```python
from build123d import *

# Parameters (mm, degrees)
F0_R     = 50.8
F1_DEPTH = 6.35
F2_DEPTH = 38.1
F3_DEPTH = 63.5


with BuildPart() as f1:
    # F0 (on Front) → F1 (new body, symmetric)
    with BuildSketch(Plane.XZ):
        Circle(F0_R)
        Polygon((0, -47.0656435661), (-38.1, 18.9254922023), (38.1, 18.9254922023), align=None, mode=Mode.SUBTRACT)
    extrude(amount=F1_DEPTH, both=True)

    # F0 (on Front) → F2 (join, symmetric)
    with BuildSketch(Plane.XZ):
        with BuildLine():
            add(Edge.make_bspline(
                [(75.8723819512, 94.9205090511), (75.9331390119, 77.3418365937), (1.5317360093, 89.0560595825), (22.3357510028, 101.1633279928)],
                knots=[0, 0, 0, 0, 53.8993844273, 53.8993844273, 53.8993844273, 53.8993844273], degree=3))
            Line((22.3357510028, 101.1633279928), (-119.3492407465, 18.707214336))
            Line((-119.3492407465, 18.707214336), (-152.3990897254, -0.5267360641))
            Line((-152.3990897254, -0.5267360641), (-119.5423719358, -19.3454558368))
            Line((-119.5423719358, -19.3454558368), (76.6557116753, -131.7181151837))
            Line((76.6557116753, -131.7181151837), (76.5361384347, -97.1223199462))
            Line((76.5361384347, -97.1223199462), (25.7361384347, -97.1223199462))
            Line((25.7361384347, -97.1223199462), (25.7361384347, -71.7223199462))
            Line((25.7361384347, -71.7223199462), (76.4483485663, -71.7223199462))
            Line((76.4483485663, -71.7223199462), (75.8723819512, 94.9205090511))
        make_face()
        Circle(F0_R, mode=Mode.SUBTRACT)
        with BuildLine():
            Line((75.7433780501, 132.2448512478), (22.3357510028, 101.1633279928))
            add(Edge.make_bspline(
                [(75.8723819512, 94.9205090511), (75.9331390119, 77.3418365937), (1.5317360093, 89.0560595825), (22.3357510028, 101.1633279928)],
                knots=[0, 0, 0, 0, 53.8993844273, 53.8993844273, 53.8993844273, 53.8993844273], degree=3))
            Line((75.8723819512, 94.9205090511), (75.7433780501, 132.2448512478))
        make_face()
        Polygon((76.5361384347, -71.7223199462), (76.4483485663, -71.7223199462), (76.5361384347, -97.1223199462), align=None)
        Polygon((76.5361384347, -97.1223199462), (76.4483485663, -71.7223199462), (25.7361384347, -71.7223199462), (25.7361384347, -97.1223199462), align=None)
    extrude(amount=F2_DEPTH, both=True)

    # F3 (add, symmetric): a face of the model
    f3_faces = [f1.faces().sort_by_distance(p)[0] for p in [
        (73.1010560932, -38.1, -114.4322968597),
    ]]
    extrude(f3_faces, amount=F3_DEPTH, both=True)


solid = f1.part
```
Can you work these out from the model? Positions are in its coordinate system, mm. A direction names the side the tool comes from. Round coordinates to 2 decimals unless told otherwise and drop trailing zeros. Order: outer loops, then holes, each group sorted by start corner. A loop starts at its lowest first (then second) coordinate and runs counter-clockwise, first axis right, second up. Notation, with made-up numbers: (18.5, 48) -> (54.5, 48) arc R21 ccw to (54.5, 59) -> close; hole circle Ø10 at (44, 2). An arc over 180 degrees is marked (long way). Return JSON: item names as keys, results as strings. Group by question number.
1. Which directions (+Z, -Z, +X, -X, +Y, -Y) give clear straight access to the entire face, cutting with the end or side of a thin tool? Please do faces 3 (the face through (-47, -101.6, 20)), 4 (the face through (-11.012, 22.447, -49.592)), 5 (the face through (-1, -6.35, 23)), 6 (the face through (-18.8, -0.1, -14.5)).
2. If we section it at C-C, the plane z = 36: Write out the boundary of the cut face in (x, y).
3. If we section it at B-B, the plane z = -24.5: Write out the boundary of the cut face in (x, y), then the cut area to 3 significant figures.
4. We'd pull the mould along Z, two halves only. Please class faces 1 (the face through (-47, 38.1, 20)), 2 (the face through (-1, 6.35, 23)): released by +Z, released by -Z, zero draft, split by the parting line, or undercut.
5. I need wall thicknesses on line 1 (X direction, y = 12.5, z = -15); line 2 (Y direction, x = -23.5, z = -44.5); line 3 (Z direction, x = 0, y = -49.5). Which ranges of each line are inside material? Lowest first, please. Write a range as [from, to].
6. If we section it at D-D, the plane x = -104: Write out the boundary of the cut face in (y, z).
7. Will these pins go through, and if not, where does the flat tip stop? pin 1 (3 mm diameter, centred on x = -18.5, y = -43.5, fed in from -Z); pin 2 (3 mm diameter, centred on x = -42.5, z = -8, fed in from +Y); pin 3 (1.5 mm diameter, centred on y = 15.5, z = 80, fed in from -X).
8. If we section it at A-A, the plane y = -78: Write out the boundary of the cut face in (x, z).
Output values:
{
 "1": {"face 3": "+Z, -Z, +X, -X, -Y", "face 4": "+Y", "face 5": "-Y", "face 6": "+Y, -Y"},
 "2": {"outline": "(-89.63, -101.6) -> (-35.84, -101.6) -> (-35.84, -6.35) -> (35.84, -6.35) -> (35.84, -101.6) -> (76.08, -101.6) -> (76.08, 38.1) -> (35.84, 38.1) -> (35.84, 6.35) -> (-35.84, 6.35) -> (-35.84, 38.1) -> (-89.63, 38.1) -> close"},
 "3": {"outline": "(-110.54, -101.6) -> (-44.5, -101.6) -> (-44.5, -6.35) -> (-13.03, -6.35) -> (-13.03, 6.35) -> (-44.5, 6.35) -> (-44.5, 38.1) -> (-110.54, 38.1) -> close; (13.03, -6.35) -> (44.5, -6.35) -> (44.5, -101.6) -> (76.29, -101.6) -> (76.29, 38.1) -> (44.5, 38.1) -> (44.5, 6.35) -> (13.03, 6.35) -> close", "area": "14,500 mm²"},
 "4": {"face 1": "zero draft", "face 2": "undercut"},
 "5": {"line 1": "[-127.13, -48.53], [48.53, 76.25]", "line 2": "[-6.35, 6.35]", "line 3": "[-87.81, -50.8], [50.8, 88.16]"},
 "6": {"outline": "(-101.6, -28.25) -> (38.1, -28.25) -> (38.1, 27.64) -> (-101.6, 27.64) -> close"},
 "7": {"pin 1": "z = -78.08", "pin 2": "y = 6.35", "pin 3": "x = -15.32"},
 "8": {"outline": "(-152.4, -0.53) -> (76.66, -131.72) -> (76.54, -97.12) -> (76.54, -71.72) -> (76.45, -71.72) -> (75.74, 132.24) -> close; hole circle Ø101.6 at (0, 0)"}
}
